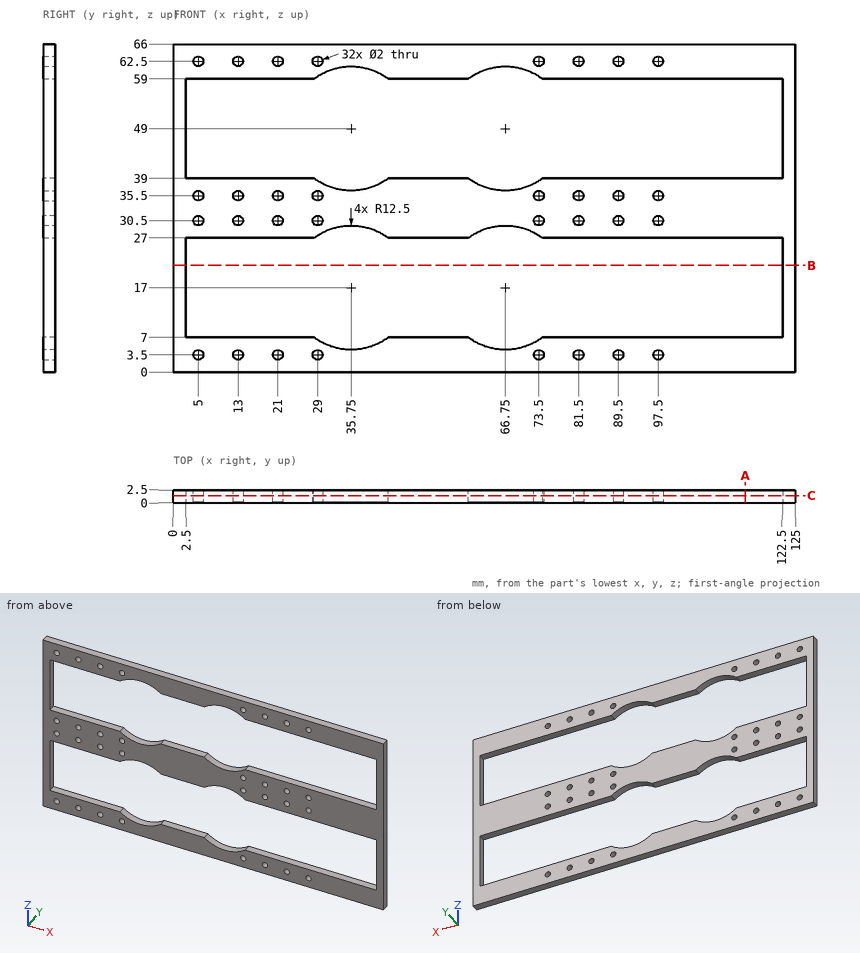
Source: three-view drawing plus pictorial views. Frame: mm from the lowest corner of the part. Round coordinates to 2 decimals unless told otherwise and drop trailing zeros. Loops run counter-clockwise (first coordinate to the right, second up) from the corner with the lowest first, then second, coordinate; pieces in that order, holes last.
Item 1: Line query: L1, parallel to Z at x = 67, y = 1.3; L2, parallel to Z at x = 44.5, y = 1.15; L3, parallel to X at y = 1.4, z = 58.5. Output: solid intervals per line, ascending.
Checked values:
L1: z = 0 to 4.5, 29.5 to 36.5, 61.5 to 66
L2: z = 0 to 7, 27 to 39, 59 to 66
L3: x = 0 to 2.5, 122.5 to 125
Item 2: Section B-B, the plane z = 21.5. Output: boundary loops of the cut face in (x, y), plus the area to 3 significant figures.
Checked values:
outline: (0, 0) - (2.5, 0) - (2.5, 2.5) - (0, 2.5) - close; (122.5, 0) - (125, 0) - (125, 2.5) - (122.5, 2.5) - close
area: 12.5 mm2
Item 3: Section C-C, the plane y = 1.4. State how many separate pieces and enclosed holes the cut face has, plus the area to 3 significant figures.
Checked values:
separate pieces: 1
enclosed holes: 34
area: 3,150 mm2
Item 4: Section A-A, the plane x = 115. Output: boundary loops of the cut face in (y, z).
Checked values:
outline: (0, 0) - (2.5, 0) - (2.5, 7) - (0, 7) - close; (0, 27) - (2.5, 27) - (2.5, 39) - (0, 39) - close; (0, 59) - (2.5, 59) - (2.5, 66) - (0, 66) - close
